Model file for the job. Use its own axes, mm. A direction names the side the tool comes from. Give positions to 0.01 mm unless a question says otherwise; leave off trailing zeros. Loops run counter-clockwise (first coordinate to the right, second up) from the corner with the lowest first, then second, coordinate; pieces in that order, holes last. Notation, with made-up numbers: (85, 19.5) - (128, 19.5) arc R26 cw to (128, 55.5) - close; hole circle Ø1 at (11, 3.25). An arc over 180 degrees is marked (long way). Use a Markdown table: item, result.
from build123d import *

# Parameters (mm, degrees)
OUTER_CASING_DEPTH  = 1.51892
SKETCH1_R           = 15
INNER_CUTOUT_DEPTH  = 20
SKETCH4_W           = 76.2
SKETCH4_H           = 1.51892
BOSS_EXTRUDE1_DEPTH = 25.4
SKETCH5_R           = 4.7625
CUT_EXTRUDE1_DEPTH  = 2.51892


with BuildPart() as part:
    # Plate shape → Outer casing (new body)
    with BuildSketch(Plane.XY):
        with BuildLine():
            Line((0, 152.4), (-152.4, 152.4))
            ThreePointArc((-152.4, 152.4), (0, 304.8), (152.4, 152.4))
            Line((152.4, 152.4), (0, 152.4))
        make_face()
    extrude(amount=OUTER_CASING_DEPTH)

    # Sketch1 → Inner Cutout (cut)
    with BuildSketch(Plane.XY.offset(1.51892)):
        with Locations((0, 152.4)):
            Circle(SKETCH1_R)
    extrude(amount=-INNER_CUTOUT_DEPTH, mode=Mode.SUBTRACT)

    # Sketch4 → Boss-Extrude1 (add)
    with BuildSketch(Plane(origin=(0, 0, 0), x_dir=(-1, 0, 0), z_dir=(0, 0, -1))):
        with Locations((-114.3, 153.15946)):
            Rectangle(SKETCH4_W, SKETCH4_H)
        with Locations((114.3, 153.15946)):
            Rectangle(SKETCH4_W, SKETCH4_H)
    extrude(amount=BOSS_EXTRUDE1_DEPTH)

    # Sketch5 → Cut-Extrude1 (cut, through all)
    with BuildSketch(Plane(origin=(0, 153.91892, 0), x_dir=(1, 0, 0), z_dir=(0, 1, 0))):
        with Locations((133.35, 12.7)):
            Circle(SKETCH5_R)
        with Locations((95.25, 12.7)):
            Circle(SKETCH5_R)
        with Locations((-133.35, 12.7)):
            Circle(SKETCH5_R)
        with Locations((-95.25, 12.7)):
            Circle(SKETCH5_R)
    extrude(amount=-CUT_EXTRUDE1_DEPTH, mode=Mode.SUBTRACT)


solid = part.part
(1) 3-axis set-ups, long thin cutter, end or side, ignore diameter. For faces 5 (the cylindrical face through (-100.008, 153.17, -12.909)), 6 (the flat face through (115, 153.919, -13)): which of +Z, -Z, +X, -X, +Y, -Y reach the whole face in a straight line?
Computed:
| item | result |
|---|---|
| face 5 | +Y, -Y |
| face 6 | -Z, +X, -X, +Y |
(2) Slice it at A-A, the plane z = -21.5. Write the cut outline in (x, y), plus the area to 3 significant figures.
Computed:
| item | result |
|---|---|
| outline | (-152.4, 152.4) - (-76.2, 152.4) - (-76.2, 153.92) - (-152.4, 153.92) - close; (76.2, 152.4) - (152.4, 152.4) - (152.4, 153.92) - (76.2, 153.92) - close |
| area | 231 mm² |
(3) Slice it at C-C, the plane x = 0. Write the cut outline in (y, z), plus the area to 3 significant figures.
Computed:
| item | result |
|---|---|
| outline | (167.4, 0) - (304.8, 0) - (304.8, 1.52) - (167.4, 1.52) - close |
| area | 209 mm² |
(4) Drill centre lines: probe 1 along X at (y, z) = (153.35, -12.7); probe 2 along Z at (x, y) = (133.35, 153.65); probe 3 along Z at (x, y) = (-133, 153). Where is each one in solid material? Low to high. Write a range as [from, to].
Computed:
| item | result |
|---|---|
| probe 1 | [-152.4, -138.11], [-128.59, -100.01], [-90.49, -76.2], [76.2, 90.49], [100.01, 128.59], [138.11, 152.4] |
| probe 2 | [-25.4, -17.46], [-7.94, 1.52] |
| probe 3 | [-25.4, -17.45], [-7.95, 1.52] |
(5) Slice it at B-B, the plane x = 133.35. Write the cut outline in (y, z).
Computed:
| item | result |
|---|---|
| outline | (152.4, -25.4) - (153.92, -25.4) - (153.92, -17.46) - (152.4, -17.46) - close; (152.4, -7.94) - (153.92, -7.94) - (153.92, 0) - (226.18, 0) - (226.18, 1.52) - (152.4, 1.52) - close |
(6) Pin check, flat tips, straight feed: P1, Ø7.5, axis at x = -95.25, z = -12.7, coming from the +Y side; P2, Ø1.5, axis at x = 58.5, y = 286, coming from the -Z side; P3, Ø7.5, axis at x = -108.5, z = -8.5, coming from the +Y side. Stop position of each tip, or through.
Computed:
| item | result |
|---|---|
| P1 | through |
| P2 | z = 0 |
| P3 | y = 153.92 |
(7) Mould opens along Z. For faces 1 (the cylindrical face through (128.592, 153.17, -12.909)), 2 (the flat face through (2, 213, 1.519)), 3 (the flat face through (2, 213, 0)), 4 (the flat face through (-114, 153.919, -13)) say: pulls with the +Z half, pulls with the -Z half, needs draft (parallel to the pull), parting line crosses it, or undercut.
Computed:
| item | result |
|---|---|
| face 1 | undercut |
| face 2 | pulls with the +Z half |
| face 3 | pulls with the -Z half |
| face 4 | needs draft |
(8) Slice it at D-D, the plane y = 258. Write the cut outline in (x, z).
Computed:
| item | result |
|---|---|
| outline | (-109.88, 0) - (109.88, 0) - (109.88, 1.52) - (-109.88, 1.52) - close |
